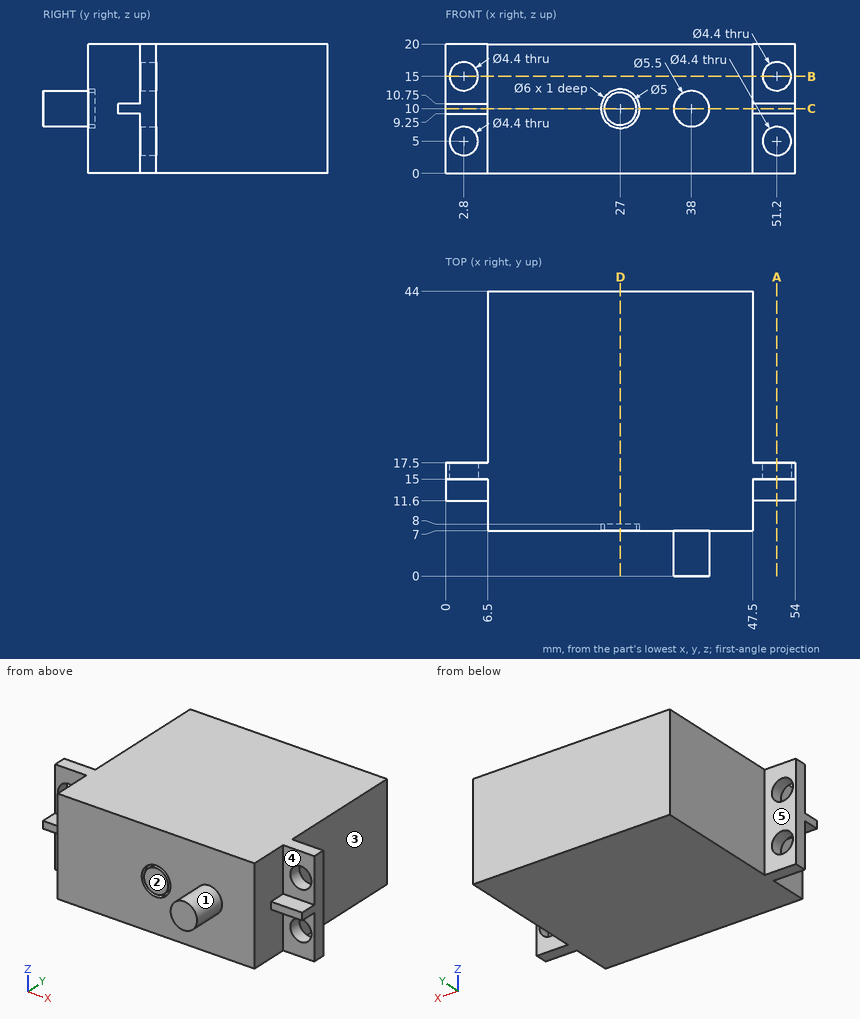
Can you work these out from the drawing? Everything is in mm from the part's minimum corner. A direction names the side the tool comes from. Coordinates: 2 decimals unless noted, no trailing zeros. Loops run counter-clockwise (first coordinate to the right, second up) from the corner with the lowest first, then second, coordinate; pieces in that order, holes last.
1) Imagine slicing it at A-A on x = 51.2. List the corners of the cut face in (y, z) for me.
2) Imagine slicing it at C-C on z = 10. List the corners of the cut face in (x, y) for me.
3) Imagine slicing it at B-B on z = 15. List the corners of the cut face in (x, y) for me.
4) I need wall thicknesses on probe 1 along Z at (x, y) = (27, 7.75); probe 2 along Z at (x, y) = (51.2, 16.8); probe 3 along X at (y, z) = (14, 1.75). Which ranges of each line are inside material? Lowest first, please.
5) Which directions (+Z, -Z, +X, -X, +Y, -Y) give clear straight access to the entire face, cutting with the end or side of a thin tool? Please do the marked faces 1, 2, 3, 4 and 5.
6) For pin 1 (7 mm diameter, centred on x = 2, z = 5, fed in from -Y); pin 2 (1.5 mm diameter, centred on y = 5, z = 8, fed in from +X); pin 3 (1.6 mm diameter, centred on x = 3.5, z = 10, fed in from -Y); pin 4 (4 mm diameter, centred on x = 51.2, z = 5, fed in from -Y), each with a flat end and sliding along its axis, tell me the tip position at first contact or that it passes through.
7) Imagine slicing it at D-D on x = 27. List the corners of the cut face in (y, z) for me.
Completed:
1. outline: (11.6, 9.25) - (15, 9.25) - (15, 7.2) - (17.5, 7.2) - (17.5, 12.8) - (15, 12.8) - (15, 10.75) - (11.6, 10.75) - close; (15, 0) - (17.5, 0) - (17.5, 2.8) - (15, 2.8) - close; (15, 17.2) - (17.5, 17.2) - (17.5, 20) - (15, 20) - close
2. outline: (0, 11.6) - (6.5, 11.6) - (6.5, 7) - (24, 7) - (24, 8) - (24.5, 8) - (24.5, 7) - (29.5, 7) - (29.5, 8) - (30, 8) - (30, 7) - (35.25, 7) - (35.25, 0) - (40.75, 0) - (40.75, 7) - (47.5, 7) - (47.5, 11.6) - (54, 11.6) - (54, 17.5) - (47.5, 17.5) - (47.5, 44) - (6.5, 44) - (6.5, 17.5) - (0, 17.5) - close
3. outline: (0, 15) - (0.6, 15) - (0.6, 17.5) - (0, 17.5) - close; (5, 15) - (6.5, 15) - (6.5, 7) - (47.5, 7) - (47.5, 15) - (49, 15) - (49, 17.5) - (47.5, 17.5) - (47.5, 44) - (6.5, 44) - (6.5, 17.5) - (5, 17.5) - close; (53.4, 15) - (54, 15) - (54, 17.5) - (53.4, 17.5) - close
4. probe 1: z = 0 to 7, 7.5 to 12.5, 13 to 20
4. probe 2: z = 0 to 2.8, 7.2 to 12.8, 17.2 to 20
4. probe 3: x = 6.5 to 47.5
5. face 1: -Y
5. face 2: +Z, -Z, -X, -Y
5. face 3: +Z, -Z, +X, +Y
5. face 4: +Z, +X, -Y
5. face 5: +Z, -Z, -X, +Y
6. pin 1: stops at y = 15
6. pin 2: stops at x = 40.45
6. pin 3: stops at y = 11.6
6. pin 4: passes through
7. outline: (7, 0) - (44, 0) - (44, 20) - (7, 20) - (7, 13) - (8, 13) - (8, 12.5) - (7, 12.5) - (7, 7.5) - (8, 7.5) - (8, 7) - (7, 7) - close
